from build123d import *

# Parameters (mm, degrees)
SKETCH1_R           = 31.75
BASE_EXTRUDE_DEPTH  = 46.99
SKETCH2_R           = 57.15
BOSS_EXTRUDE1_DEPTH = 19.05
SKETCH4_R           = 47.625
CUT_EXTRUDE1_DEPTH  = 12.7
CUT_EXTRUDE2_DEPTH  = 105.372058521


with BuildPart() as part:
    # Sketch1 → Base-Extrude (new body)
    with BuildSketch(Plane.XY):
        Circle(SKETCH1_R)
    extrude(amount=-BASE_EXTRUDE_DEPTH)

    # Sketch2 → Boss-Extrude1 (add)
    with BuildSketch(Plane(origin=(0, 0, -46.99), x_dir=(-1, 0, 0), z_dir=(0, 0, -1))):
        Circle(SKETCH2_R)
    extrude(amount=BOSS_EXTRUDE1_DEPTH)

    # Sketch4 → Cut-Extrude1 (cut)
    with BuildSketch(Plane(origin=(0, 0, -66.04), x_dir=(-1, 0, 0), z_dir=(0, 0, -1))):
        Circle(SKETCH4_R)
    extrude(amount=-CUT_EXTRUDE1_DEPTH, mode=Mode.SUBTRACT)

    # Sketch6 → Cut-Extrude2 (cut, through all)
    with BuildSketch(Plane.XY):
        with BuildLine():
            Line((-3.175, 12.065), (3.175, 12.065))
            Line((3.175, 12.065), (3.175, 8.980256121))
            ThreePointArc((3.175, 8.980256121), (0, -9.525), (-3.175, 8.980256121))
            Line((-3.175, 8.980256121), (-3.175, 12.065))
        make_face()
    extrude(amount=-CUT_EXTRUDE2_DEPTH, mode=Mode.SUBTRACT)


solid = part.part
The model under review builds one solid part; all positions refer to its coordinate system, in mm. A direction names the side the tool comes from. Round coordinates to 2 decimals unless told otherwise and drop trailing zeros. Write each loop counter-clockwise with the first axis right and the second up, starting at its lowest first coordinate (ties: lowest second). Pieces come first, ordered by that corner, then holes. Notation, with made-up numbers: (6.25, 71) - (40.25, 71) arc R23 cw to (40.25, 102) - close; hole circle Ø1 at (67, -13.75). An arc over 180 degrees is marked (long way). One line per item, written item: value. Start each with the question number.
1. Consider section C-C on z = -19.5. Write out the cut boundary in (x, y) (3 decimals).
2. The part is to be moulded in two halves that separate along X. For faces 5 (the face through (21, 43, -66.04)), 6 (the face through (-3.175, 11, -26)), 7 (the face through (-6.883, -30.995, -23.166)), 8 (the face through (37.794, -28.979, -59.779)), say which applies: released by +X, released by -X, zero draft, split by the parting line, or undercut.
3. Clearance check with flat-ended pins moving along their axes: P1, Ø3, axis at x = 1.5, z = -30, coming from the -Y side; P2, Ø3.5, axis at y = 10.5, z = -16.5, coming from the -X side; P3, Ø12, axis at y = -14, z = -37, coming from the +X side. State where each tip first meets the part, or that it passes through.
4. Consider section B-B on y = 0. Write out the cut boundary in (x, z) (3 decimals).
5. Consider section A-A on x = 0. Write out the cut boundary in (y, z) (3 decimals).
6. To check wall thickness, follow L1, parallel to Z at x = -18, y = -6; L2, parallel to Z at x = -39, y = 37.5; L3, parallel to X at y = 12, z = -33 (3 decimals). State the ranges of each line that lie inside material, in increasing order. Write a range as from..to.
7. Consider section D-D on x = -21. Write out the cut boundary in (y, z).
8. Machinability: for faces 1 (the face through (7, 8, 0)), 2 (the face through (-25, -25, -46.99)), 3 (the face through (0, 12.065, -26)), 4 (the face through (1, -10, -53.34)), which of the approach directions +Z, -Z, +X, -X, +Y, -Y give a long, thin tool a straight path to every point of the face, cutting with its end or side? Answer none if there is none.
Checks:
1. outline: circle Ø63.5 at (0, 0); hole (-3.175, 8.98) arc R9.525 ccw (long way) to (3.175, 8.98) - (3.175, 12.065) - (-3.175, 12.065) - close
2. face 5: zero draft
2. face 6: undercut
2. face 7: split by the parting line
2. face 8: undercut
3. P1: stops at y = -31.75
3. P2: stops at x = -30.52
3. P3: stops at x = 30.73
4. outline: (-57.15, -66.04) - (-47.625, -66.04) - (-47.625, -53.34) - (-9.525, -53.34) - (-9.525, 0) - (-31.75, 0) - (-31.75, -46.99) - (-57.15, -46.99) - close; (9.525, -53.34) - (47.625, -53.34) - (47.625, -66.04) - (57.15, -66.04) - (57.15, -46.99) - (31.75, -46.99) - (31.75, 0) - (9.525, 0) - close
5. outline: (-57.15, -66.04) - (-47.625, -66.04) - (-47.625, -53.34) - (-9.525, -53.34) - (-9.525, 0) - (-31.75, 0) - (-31.75, -46.99) - (-57.15, -46.99) - close; (12.065, -53.34) - (47.625, -53.34) - (47.625, -66.04) - (57.15, -66.04) - (57.15, -46.99) - (31.75, -46.99) - (31.75, 0) - (12.065, 0) - close
6. L1: z = -53.34..0
6. L2: z = -66.04..-46.99
6. L3: x = -29.395..-3.175, 3.175..29.395
7. outline: (-53.15, -66.04) - (-42.75, -66.04) - (-42.75, -53.34) - (42.75, -53.34) - (42.75, -66.04) - (53.15, -66.04) - (53.15, -46.99) - (23.81, -46.99) - (23.81, 0) - (-23.81, 0) - (-23.81, -46.99) - (-53.15, -46.99) - close
8. face 1: +Z, +X, -X, +Y, -Y
8. face 2: +Z
8. face 3: +Z, -Z
8. face 4: -Z
